Check sheet for the drawn part. Datum: minimum x, y, z corner. Units: mm. A direction names the side the tool comes from. Give positions to 0.01 mm unless a question says otherwise; leave off trailing zeros. Loops run counter-clockwise (first coordinate to the right, second up) from the corner with the lowest first, then second, coordinate; pieces in that order, holes last. Notation, with made-up numbers: (32.5, 84) - (55.5, 84) arc R25 ccw to (55.5, 121) - close; hole circle Ø2 at (59, 66.5). An arc over 180 degrees is marked (long way). Use one line per item in the form item = value.
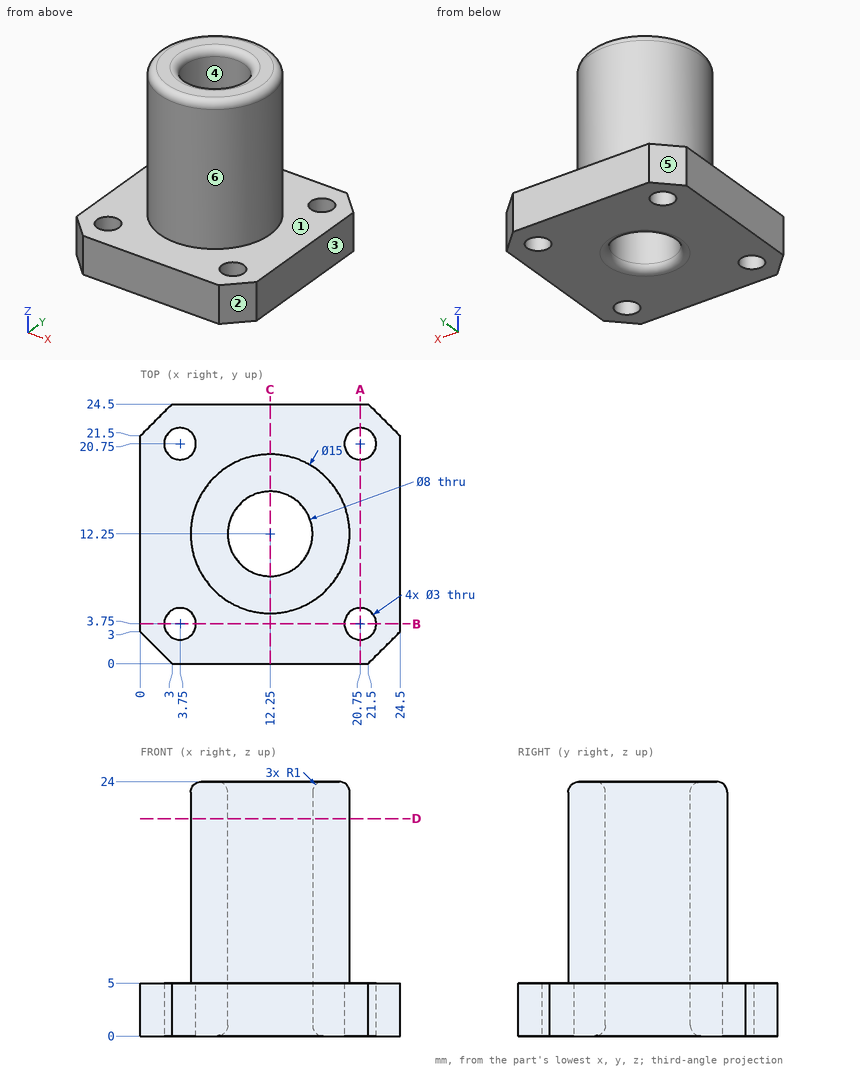
Item 1: Access from +Z, -Z, +X, -X, +Y, -Y to the whole of each face (thin tool, end or side, straight path). Record for the marked faces 1 and 2.
Answer block:
face_1 = +Z
face_2 = +Z, -Z, +X, -Y
Item 2: Thickness scan on L1, parallel to Y at x = 3.75, z = 1.55; L2, parallel to X at y = 12, z = 5.25; L3, parallel to Z at x = 4.25, y = 23.75. Record the ranges inside material, lowest first.
Answer block:
L1 = 0 to 2.25, 5.25 to 19.25, 22.25 to 24.5
L2 = 4.75 to 8.26, 16.24 to 19.75
L3 = 0 to 5
Item 3: Section check D-D on z = 20.5. Record the boundary of the cut face in (x, y).
Answer block:
outline = circle Ø15 at (12.25, 12.25); hole circle Ø8 at (12.25, 12.25)
Item 4: Mould release check, pull along Y, two halves, no side actions. Record for the marked faces 3, 4, 5 and 6: released by +Y, released by -Y, zero draft, split by the parting line, or undercut.
Answer block:
face_3 = zero draft
face_4 = undercut
face_5 = released by +Y
face_6 = split by the parting line
Item 5: Section check A-A on x = 20.75. Record the boundary of the cut face in (y, z).
Answer block:
outline = (0, 0) - (2.25, 0) - (2.25, 5) - (0, 5) - close; (5.25, 0) - (19.25, 0) - (19.25, 5) - (5.25, 5) - close; (22.25, 0) - (24.5, 0) - (24.5, 5) - (22.25, 5) - close
Item 6: Section check C-C on x = 12.25. Record the boundary of the cut face in (y, z).
Answer block:
outline = (0, 0) - (7.25, 0) arc R1 ccw to (8.25, 1) - (8.25, 23) arc R1 ccw to (7.25, 24) - (5.75, 24) arc R1 ccw to (4.75, 23) - (4.75, 5) - (0, 5) - close; (16.25, 1) arc R1 ccw to (17.25, 0) - (24.5, 0) - (24.5, 5) - (19.75, 5) - (19.75, 23) arc R1 ccw to (18.75, 24) - (17.25, 24) arc R1 ccw to (16.25, 23) - close
Item 7: Gauge pin test, flat ends, axial feed: P1, Ø2.5, axis at x = 3.75, y = 20.75, coming from the +Z side; P2, Ø8, axis at x = 14.5, z = 13.5, coming from the -Y side; P3, Ø2, axis at y = 15.5, z = 14.5, coming from the -X side; P4, Ø1, axis at x = 8, y = 6.5, coming from the +Z side. Record the tip position at first contact, or that the pin passes through.
Answer block:
P1 = through
P2 = 4.75
P3 = 5.1
P4 = 23.99
